```python
from build123d import *

# Parameters (mm, degrees)
F0_W     = 27.5
F0_H     = 47
F1_DEPTH = 18
F0_W_2   = 30.5
F0_H_2   = 50
F2_DEPTH = 3


with BuildPart() as f1:
    # F0 (on Top) → F1 (new body)
    with BuildSketch(Plane.XY):
        Rectangle(F0_W, F0_H)
    extrude(amount=F1_DEPTH)

    # F0 (on Top) → F2 (join)
    with BuildSketch(Plane.XY):
        Rectangle(F0_W_2, F0_H_2)
        Rectangle(F0_W, F0_H, mode=Mode.SUBTRACT)
        Rectangle(F0_W, F0_H)
    extrude(amount=-F2_DEPTH)


solid = f1.part
```
Source: CAD feature listing. Evaluate the final solid. Frame: model axes, mm. A direction names the side the tool comes from. Coordinates: 2 decimals unless noted, no trailing zeros. Loops run counter-clockwise (first coordinate to the right, second up) from the corner with the lowest first, then second, coordinate; pieces in that order, holes last. Notation, with made-up numbers: M -19,64.5 L -4,64.5 A13 cw -4,84.5 Z; hole C 22.25,29 d7. An arc over 180 degrees is marked long. Use a Markdown table: item, result. Add a question column.
Q1. Material intervals for L1, parallel to X at y = -18.5, z = 13.5; L2, parallel to Y at x = 11, z = 6; L3, parallel to Z at x = -14, y = -21, sorted ascending.
Q2. Section query A-A, the plane x = -4. Return loops of the section in (y, z).
Q3. First-contact query: pin 1 (4 mm diameter, centred on y = 16, z = 8, fed in from +X); pin 2 (5 mm diameter, centred on x = -9, z = 4, fed in from +Y); pin 3 (2 mm diameter, centred on y = 19, z = 11, fed in from -X). Flat tips, straight axial feed; report the tip coordinate or a pass-through.
Q4. Access query for faces 1 (the flat face through (0, -23.5, 9)), 2 (the flat face through (0, 23.5, 9)), 3 (the flat face through (13.75, 0, 9)), 4 (the flat face through (-13.75, 0, 9)). Directions: +Z, -Z, +X, -X, +Y, -Y. A direction counts if a zero-diameter tool reaches every point of the face in a straight line with its end or side. Return the directions, or none.
Q5. Section query C-C, the plane z = 1. Return loops of the section in (x, y), and give its area (3 significant figures).
Q6. Section query B-B, the plane y = 4. Return loops of the section in (x, z).
Result:
| question | item | result |
|---|---|---|
| 1 | L1 | x = -13.75 to 13.75 |
| 1 | L2 | y = -23.5 to 23.5 |
| 1 | L3 | z = -3 to 0 |
| 2 | outline | M -25,-3 L 25,-3 L 25,0 L 23.5,0 L 23.5,18 L -23.5,18 L -23.5,0 L -25,0 Z |
| 3 | pin 1 | stops at x = 13.75 |
| 3 | pin 2 | stops at y = 23.5 |
| 3 | pin 3 | stops at x = -13.75 |
| 4 | face 1 | +Z, +X, -X, -Y |
| 4 | face 2 | +Z, +X, -X, +Y |
| 4 | face 3 | +Z, +X, +Y, -Y |
| 4 | face 4 | +Z, -X, +Y, -Y |
| 5 | outline | M -13.75,-23.5 L 13.75,-23.5 L 13.75,23.5 L -13.75,23.5 Z |
| 5 | area | 1,290 mm2 |
| 6 | outline | M -15.25,-3 L 15.25,-3 L 15.25,0 L 13.75,0 L 13.75,18 L -13.75,18 L -13.75,0 L -15.25,0 Z |
